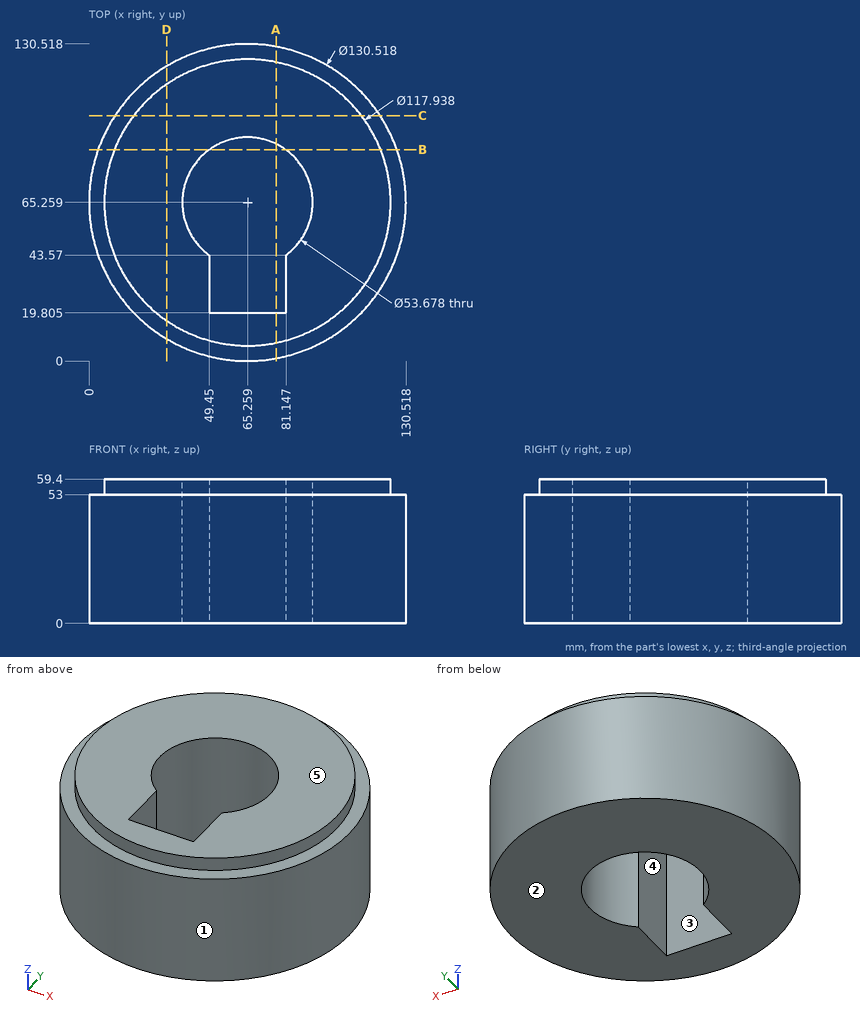
Print and shaded views of the part. All mm, measured from the part's lowest x, y and z. A direction names the side the tool comes from. Round coordinates to 2 decimals unless told otherwise and drop trailing zeros. Write each loop counter-clockwise with the first axis right and the second up, starting at its lowest first coordinate (ties: lowest second). Pieces come first, ordered by that corner, then holes. Notation, with made-up numbers: (-13.75, -5) -> (43.25, -5) arc R35 cw to (43.25, 33) -> close; hole circle Ø9 at (7, 28.5). An arc over 180 degrees is marked (long way). Return JSON: item names as keys, results as strings. Group by question number.
Q1. Saw through at C-C on y = 101. Write the cut outline in (x, z) (1 decimal).
Q2. Mould opens along X. For the marked faces 1, 2 and 3 say: pulls with the +X half, pulls with the -X half, needs draft (parallel to the pull), parting line crosses it, or undercut.
Q3. Saw through at D-D on x = 32. Write the cut outline in (y, z).
Q4. Saw through at A-A on x = 77. Write the cut outline in (y, z) (1 decimal), plus the area to 3 significant figures.
Q5. Probe L1, parallel to X at y = 26, z = 17.5; L2, parallel to X at y = 52, z = 43 (1 decimal); L3, parallel to Y at x = 60.5, z = 39.5 (1 decimal). List the from-to ranges inside material, lowest first. Write a range as [from, to].
Q6. Saw through at B-B on y = 87. Write the cut outline in (x, z) (1 decimal).
Q7. Which spindle directions (+Z, -Z, +X, -X, +Y, -Y) get a long thin tool onto all of the face, cutting with end or side? Do the marked faces 4 and 5. Say none if no direction does.
Q8. Pin check, flat tips, straight feed: pin 1 (12 mm diameter, centred on y = 32, z = 42, fed in from +X); pin 2 (10 mm diameter, centred on x = 80, z = 16, fed in from +Y); pin 3 (4 mm diameter, centred on x = 99, z = 6, fed in from -Y). Stop position of each tip, or through.
Answer:
{
 "1": {"outline": "(10.7, 0) -> (119.9, 0) -> (119.9, 53) -> (112.2, 53) -> (112.2, 59.4) -> (18.4, 59.4) -> (18.4, 53) -> (10.7, 53) -> close"},
 "2": {"face 1": "parting line crosses it", "face 2": "needs draft", "face 3": "undercut"},
 "3": {"outline": "(9.11, 0) -> (121.41, 0) -> (121.41, 53) -> (113.95, 53) -> (113.95, 59.4) -> (16.56, 59.4) -> (16.56, 53) -> (9.11, 53) -> close"},
 "4": {"outline": "(1.1, 0) -> (19.8, 0) -> (19.8, 59.4) -> (7.5, 59.4) -> (7.5, 53) -> (1.1, 53) -> close; (89.4, 0) -> (129.5, 0) -> (129.5, 53) -> (123, 53) -> (123, 59.4) -> (89.4, 59.4) -> close", "area": "3,410 mm2"},
 "5": {"L1": "[13.13, 49.45], [81.15, 117.39]", "L2": "[1.4, 41.9], [88.6, 129.2]", "L3": "[0.2, 19.8], [91.7, 130.3]"},
 "6": {"outline": "(3.7, 0) -> (49.5, 0) -> (49.5, 59.4) -> (10.4, 59.4) -> (10.4, 53) -> (3.7, 53) -> close; (81, 0) -> (126.8, 0) -> (126.8, 53) -> (120.1, 53) -> (120.1, 59.4) -> (81, 59.4) -> close"},
 "7": {"face 4": "+Z, -Z", "face 5": "+Z, +X, -X, +Y, -Y"},
 "8": {"pin 1": "x = 124.55", "pin 2": "y = 129.79", "pin 3": "y = 8.24"}
}
